Could you check a few things on this model? Use its own coordinates, in mm. A direction names the side the tool comes from. Give positions to 0.01 mm unless a question says otherwise; leave off trailing zeros. Order: outer loops, then holes, each group sorted by start corner. A loop starts at its lowest first (then second) coordinate and runs counter-clockwise, first axis right, second up. Notation, with made-up numbers: M 5.25,52.5 L 18.25,52.5 A20 cw 18.25,75.5 Z; hole C 76.25,4 d3. An arc over 180 degrees is marked long. Use a Markdown table: item, result. Add a question column.
```python
from build123d import *

# Parameters (mm, degrees)
SKETCH_1_W                       = 30
SKETCH_1_H                       = 35
EXTRUDE_1_DEPTH                  = 0.75
SKETCH_2_R                       = 1.05
CUT_EXTRUDE_1_DEPTH              = 1.5
EXTRUDE_2_DEPTH                  = 2.1
SKETCH_4_W                       = 7.3
SKETCH_4_H                       = 3.5
EXTRUDE_3_DEPTH                  = 5
SKETCH_5_W                       = 7.3
SKETCH_5_H                       = 3.5
EXTRUDE_4_DEPTH                  = 5
PATTERN_LINEAR_1_COUNT           = 2
PATTERN_LINEAR_1_PITCH           = 9
PATTERN_LINEAR_2_COUNT           = 3
PATTERN_LINEAR_2_PITCH           = 8
PATTERN_LINEAR_2_COPY_1_SKETCH_W = 7.3
PATTERN_LINEAR_2_COPY_1_SKETCH_H = 3.5
PATTERN_LINEAR_2_COPY_1_DEPTH    = 5
PATTERN_LINEAR_2_COPY_2_SKETCH_W = 7.3
PATTERN_LINEAR_2_COPY_2_SKETCH_H = 3.5
PATTERN_LINEAR_2_COPY_2_DEPTH    = 5
SKETCH_6_W                       = 3
SKETCH_6_H                       = 8
EXTRUDE_5_DEPTH                  = 4.5
SKETCH_7_W                       = 8
SKETCH_7_H                       = 20
EXTRUDE_6_DEPTH                  = 10
SKETCH_8_W                       = 5.5
SKETCH_8_H                       = 10
EXTRUDE_7_DEPTH                  = 8


with BuildPart() as part:
    # ｽｹｯﾁ1 → ﾎﾞｽ - 押し出し1 (new, symmetric)
    with BuildSketch(Plane(origin=(0, 0, 0), x_dir=(1, 0, 0), z_dir=(0, 1, 0))):
        Rectangle(SKETCH_1_W, SKETCH_1_H)
    extrude(amount=EXTRUDE_1_DEPTH, both=True)

    # ｽｹｯﾁ2 → ｶｯﾄ - 押し出し1 (cut)
    with BuildSketch(Plane.XZ.offset(0.75)):
        with Locations(Location((-12.5, 15, 0), (0, 0, 270))):
            Circle(SKETCH_2_R)
        with Locations(Location((-12.5, -15, 0), (0, 0, 270))):
            Circle(SKETCH_2_R)
        with Locations(Location((12.5, 15, 0), (0, 0, 270))):
            Circle(SKETCH_2_R)
        with Locations(Location((12.5, -15, 0), (0, 0, 270))):
            Circle(SKETCH_2_R)
    extrude(amount=-CUT_EXTRUDE_1_DEPTH, mode=Mode.SUBTRACT)

    # ｽｹｯﾁ3 → ﾎﾞｽ - 押し出し2 (add)
    with BuildSketch(Plane.XZ.offset(0.75)):
        Polygon((-10, 17.5), (-10, 13.5), (-15, 13.5), (-15, -12.5), (-10, -12.5), (-10, -17.5), (10, -17.5), (10, -12.5), (15, -12.5), (15, 12.5), (10, 12.5), (10, 17.5), align=None)
    extrude(amount=EXTRUDE_2_DEPTH)

    # ｽｹｯﾁ4 → ﾎﾞｽ - 押し出し3 (add)
    with BuildSketch(Plane(origin=(0, 0.75, 0), x_dir=(1, 0, 0), z_dir=(0, 1, 0))):
        with Locations((5.85, -14.75)):
            Rectangle(SKETCH_4_W, SKETCH_4_H)
    extrude(amount=EXTRUDE_3_DEPTH)

    # ｽｹｯﾁ5 → ﾎﾞｽ - 押し出し4 (add)
    with BuildSketch(Plane(origin=(0, 0.75, 0), x_dir=(1, 0, 0), z_dir=(0, 1, 0))):
        with Locations((-10.35, 11.25)):
            Rectangle(SKETCH_5_W, SKETCH_5_H)
    extrude_4 = extrude(amount=EXTRUDE_4_DEPTH)

    # 直線ﾊﾟﾀｰﾝ1: ﾎﾞｽ - 押し出し4 ×2
    with Locations(*[(i * PATTERN_LINEAR_1_PITCH, 0, 0) for i in range(1, PATTERN_LINEAR_1_COUNT)]):
        add(extrude_4)

    # 直線ﾊﾟﾀｰﾝ2: ﾎﾞｽ - 押し出し4 ×3
    with Locations(*[(0, 0, i * PATTERN_LINEAR_2_PITCH) for i in range(1, PATTERN_LINEAR_2_COUNT)]):
        add(extrude_4)

    # 直線ﾊﾟﾀｰﾝ2 copy 1 sketch → 直線ﾊﾟﾀｰﾝ2 copy 1 (add)
    with BuildSketch(Plane(origin=(9, 0.75, 8), x_dir=(1, 0, 0), z_dir=(0, 1, 0))):
        with Locations((-10.35, 11.25)):
            Rectangle(PATTERN_LINEAR_2_COPY_1_SKETCH_W, PATTERN_LINEAR_2_COPY_1_SKETCH_H)
    extrude(amount=PATTERN_LINEAR_2_COPY_1_DEPTH)

    # 直線ﾊﾟﾀｰﾝ2 copy 2 sketch → 直線ﾊﾟﾀｰﾝ2 copy 2 (add)
    with BuildSketch(Plane(origin=(9, 0.75, 16), x_dir=(1, 0, 0), z_dir=(0, 1, 0))):
        with Locations((-10.35, 11.25)):
            Rectangle(PATTERN_LINEAR_2_COPY_2_SKETCH_W, PATTERN_LINEAR_2_COPY_2_SKETCH_H)
    extrude(amount=PATTERN_LINEAR_2_COPY_2_DEPTH)

    # ｽｹｯﾁ6 → ﾎﾞｽ - 押し出し5 (add)
    with BuildSketch(Plane(origin=(0, 0.75, 0), x_dir=(1, 0, 0), z_dir=(0, 1, 0))):
        with Locations((12.5, 6.5)):
            Rectangle(SKETCH_6_W, SKETCH_6_H)
    extrude(amount=EXTRUDE_5_DEPTH)

    # ｽｹｯﾁ7 → ﾎﾞｽ - 押し出し6 (add)
    with BuildSketch(Plane(origin=(0, 0.75, 0), x_dir=(1, 0, 0), z_dir=(0, 1, 0))):
        with Locations((-6, -21.5)):
            Rectangle(SKETCH_7_W, SKETCH_7_H)
    extrude(amount=EXTRUDE_6_DEPTH)

    # ｽｹｯﾁ8 → ﾎﾞｽ - 押し出し7 (add)
    with BuildSketch(Plane(origin=(0, 0.75, 0), x_dir=(1, 0, 0), z_dir=(0, 1, 0))):
        with Locations((6.75, 11)):
            Rectangle(SKETCH_8_W, SKETCH_8_H)
    extrude(amount=EXTRUDE_7_DEPTH)


solid = part.part
```
1) For faces 5 (the face through (-6.7, 3, -11)), 6 (the face through (-1, 3, 6.5)), 7 (the face through (-6, 0.75, 24)), 8 (the face through (-14, -0.75, -15)), which set-ups out of +Z, -Z, +X, -X, +Y, -Y let a thin tool reach every point of the face, with its end or its side?
2) Suppose I cut it at B-B on x = 12.5. Please give me the cut outline in (y, z), and give its area (3 significant figures).
3) Suppose I cut it at A-A on z = -15. Please give me the cut outline in (x, y).
4) Please list where these lines run through material, in increasing order: line 1 (X direction, y = 0, z = 15); line 2 (Z direction, x = 5.5, y = 1.75); line 3 (X direction, y = 2, z = -9). Write a range as from..to.
5) Suppose I cut it at C-C on x = 3.5. Please give me the cut outline in (y, z), and give its area (4 significant figures).
6) Suppose I cut it at D-D on z = 15. Please give me the cut outline in (x, y).
7) For pin 1 (4 mm diameter, centred on x = 5, y = 3, fed in from -Z); pin 2 (5.5 mm diameter, centred on x = 7, y = 4, fed in from +Z); pin 3 (1 mm diameter, centred on x = 12.5, y = -2, fed in from +Z); pin 4 (3 mm diameter, centred on y = 8, z = -0.5, fed in from +X), each with a flat end and sliding along its axis, tell me the tip position at first contact or that it passes through.
8) We'd pull the mould along X, two halves only. Please class faces 1 (the face through (4, 5, -11)), 2 (the face through (-14, 3, -3)), 3 (the face through (-5, 3, -11)), 4 (the face through (-10, 3, 6.5)): pulls with the +X half, pulls with the -X half, needs draft (parallel to the pull), parting line crosses it, or undercut.
Values found:
| question | item | result |
|---|---|---|
| 1 | face 5 | -Z, +Y |
| 1 | face 6 | +X, -X, +Y |
| 1 | face 7 | +Z, +X, -X, -Y |
| 1 | face 8 | -Z, -X, -Y |
| 2 | outline | M -2.85,-12.5 L -0.75,-12.5 L -0.75,-13.95 L 0.75,-13.95 L 0.75,-10.5 L 5.25,-10.5 L 5.25,-2.5 L 0.75,-2.5 L 0.75,13.95 L -0.75,13.95 L -0.75,12.5 L -2.85,12.5 Z; M -0.75,-17.5 L 0.75,-17.5 L 0.75,-16.05 L -0.75,-16.05 Z; M -0.75,16.05 L 0.75,16.05 L 0.75,17.5 L -0.75,17.5 Z |
| 2 | area | 135 mm^2 |
| 3 | outline | M -15,-0.75 L -13.55,-0.75 L -13.55,0.75 L -15,0.75 Z; M -11.45,-0.75 L -10,-0.75 L -10,-2.85 L 10,-2.85 L 10,-0.75 L 11.45,-0.75 L 11.45,0.75 L 9.5,0.75 L 9.5,8.75 L 4,8.75 L 4,0.75 L -11.45,0.75 Z; M 13.55,-0.75 L 15,-0.75 L 15,0.75 L 13.55,0.75 Z |
| 4 | line 1 | x = -15..-13.55, -11.45..11.45, 13.55..15 |
| 4 | line 2 | z = -16..-6, 13..16.5 |
| 4 | line 3 | x = 4..9.5, 11..14 |
| 5 | outline | M -2.85,-17.5 L 0.75,-17.5 L 0.75,13 L 5.75,13 L 5.75,16.5 L 0.75,16.5 L 0.75,17.5 L -2.85,17.5 Z |
| 5 | area | 143.5 mm^2 |
| 6 | outline | M -15,-0.75 L -13.55,-0.75 L -13.55,0.75 L -15,0.75 Z; M -11.45,-0.75 L -10,-0.75 L -10,-2.85 L 10,-2.85 L 10,-0.75 L 11.45,-0.75 L 11.45,0.75 L 9.5,0.75 L 9.5,5.75 L 2.2,5.75 L 2.2,0.75 L -2,0.75 L -2,10.75 L -10,10.75 L -10,0.75 L -11.45,0.75 Z; M 13.55,-0.75 L 15,-0.75 L 15,0.75 L 13.55,0.75 Z |
| 7 | pin 1 | stops at z = -16 |
| 7 | pin 2 | stops at z = 16.5 |
| 7 | pin 3 | stops at z = 12.5 |
| 7 | pin 4 | passes through |
| 8 | face 1 | undercut |
| 8 | face 2 | pulls with the -X half |
| 8 | face 3 | undercut |
| 8 | face 4 | needs draft |
